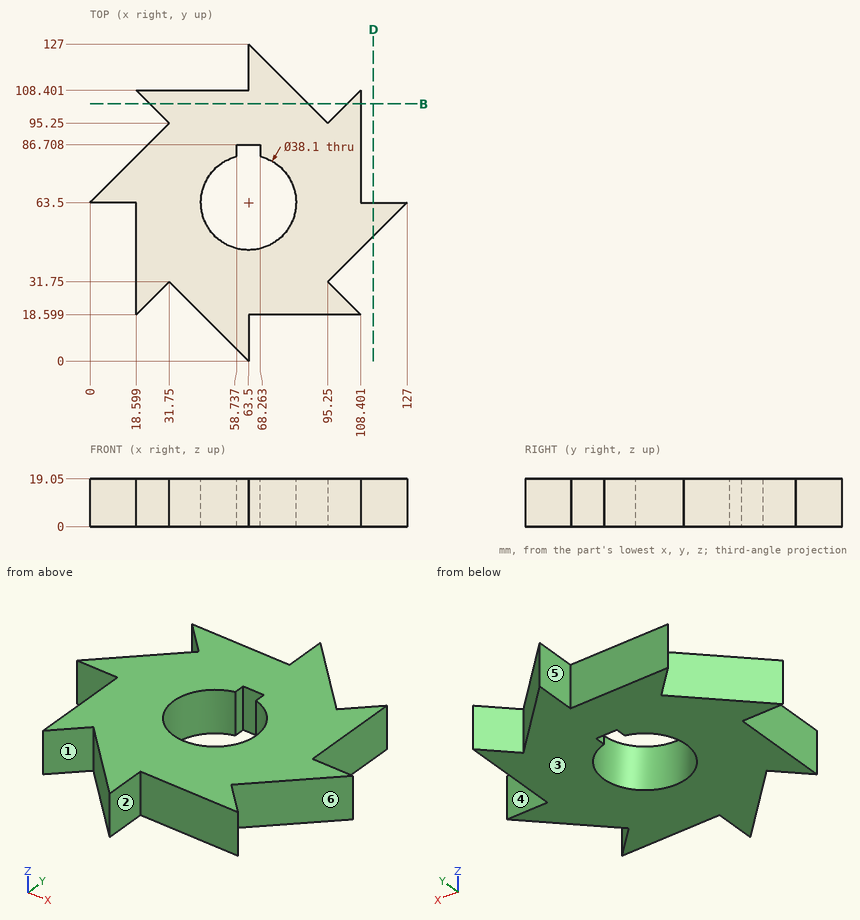
Can you work these out from the drawing? Everything is in mm from the part's minimum corner. A direction names the side the tool comes from. Give positions to 0.01 mm unless a question says otherwise; leave off trailing zeros. Order: outer loops, then holes, each group sorted by start corner. A loop starts at its lowest first (then second) coordinate and runs counter-clockwise, first axis right, second up. Notation, with made-up numbers: M 85,74.25 L 135,74.25 A33 cw 135,103.25 Z; hole C -18.5,44.5 d1. An arc over 180 degrees is marked long. Use a Markdown table: item, result. Add a question column.
Item 1: We'd pull the mould along X, two halves only. Please class the marked faces 1, 2 and 3: +X half, -X half, draft (parallel to the pull), parting line (faces both ways), or undercut.
Item 2: Will these pins go through, and if not, where does the flat tip stop? pin 1 (8 mm diameter, centred on x = 101.5, z = 13.5, fed in from -Y); pin 2 (3 mm diameter, centred on x = 98, y = 86.5, fed in from -Z); pin 3 (9.5 mm diameter, centred on x = 34, z = 10.5, fed in from +Y); pin 4 (1.4 mm diameter, centred on y = 84.5, z = 5.5, fed in from -X).
Item 3: If I drill on L1, parallel to Y at x = 104.5, z = 10; L2, parallel to Y at x = 61.5, z = 2 (1 decimal); L3, parallel to X at y = 58, z = 15.5, over which ranges is the centre line in solid material (lowest first)? Write a range as [from, to].
Item 4: Suppose I cut it at D-D (x = 113.5). List the corners of the cut face in (y, z) for me.
Item 5: Suppose I cut it at B-B (y = 103). List the corners of the cut face in (x, z) for me, then the cut area to 3 significant figures.
Item 6: For the marked faces 4, 5 and 6, which set-ups out of +Z, -Z, +X, -X, +Y, -Y let a thin tool reach every point of the face, with its end or its side?
Answer sheet:
| question | item | result |
|---|---|---|
| 1 | face 1 | undercut |
| 1 | face 2 | +X half |
| 1 | face 3 | draft |
| 2 | pin 1 | stops at y = 18.6 |
| 2 | pin 2 | stops at z = 0 |
| 2 | pin 3 | stops at y = 108.4 |
| 2 | pin 4 | stops at x = 20.3 |
| 3 | L1 | y = [18.6, 22.5], [41, 104.5] |
| 3 | L2 | y = [2, 44.6], [86.7, 108.4] |
| 3 | L3 | x = [18.6, 45.26], [81.74, 121.5] |
| 4 | outline | M 50,0 L 63.5,0 L 63.5,19.05 L 50,19.05 Z |
| 5 | outline | M 24,0 L 87.5,0 L 87.5,19.05 L 24,19.05 Z; M 103,0 L 108.4,0 L 108.4,19.05 L 103,19.05 Z |
| 5 | area | 1,310 mm² |
| 6 | face 4 | +Z, -Z, +X, +Y |
| 6 | face 5 | +Z, -Z, -X, +Y |
| 6 | face 6 | +Z, -Z, +X |
